The model under review builds one solid part; all positions refer to its coordinate system, in mm. Round coordinates to 2 decimals unless told otherwise and drop trailing zeros. Write each loop counter-clockwise with the first axis right and the second up, starting at its lowest first coordinate (ties: lowest second). Pieces come first, ordered by that corner, then holes. Notation, with made-up numbers: M -10.75,-17.75 L 23.25,-17.75 A21 ccw 23.25,12.25 Z; hole C 61.5,15.25 d8. An arc over 180 degrees is marked long. One line per item, written item: value. Start each with the question number.
1) Take a section at B-B, the plane x = 35. Write out the cut boundary in (y, z), and give its area (3 significant figures).
2) Take a section at A-A, the plane y = 12. Write out the cut boundary in (x, z), and give its area (3 significant figures).
3) Take a section at D-D, the plane z = 0. Write out the cut boundary in (x, y).
4) Take a section at C-C, the plane z = -35. Write out the cut boundary in (x, y).
5) For P1, Ø1, axis at x = -38.5, z = -12.5, coming from the +Y side; P2, Ø12, axis at y = 5, z = -22.5, coming from the +X side; P3, Ø12, axis at y = 13.5, z = -32, coming from the +X side, all flat-tipped, find the tip position at first contact; note any pin that passes through.
6) Wall thickness on probe 1 along Y at (x, z) = (41.5, -6.5); probe 2 along X at (y, z) = (5.5, -20); probe 3 along Z at (x, y) = (33, 16.5): over which ranges is each line inside the solid? List them lowest first.
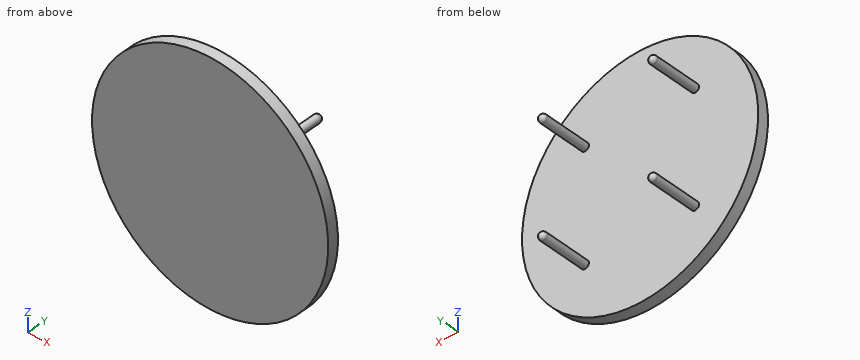
from build123d import *

# Parameters (mm, degrees)
SKETCH1_R                      = 75
BOSS_EXTRUDE1_DEPTH            = 7
SKETCH2_R                      = 2.5
BOSS_EXTRUDE2_DEPTH            = 30
DOME1_FACE_RADIUS              = 2.5
DOME1_HEIGHT                   = 2.5
CIRPATTERN1_COUNT              = 4
CIRPATTERN1_COPY_1_FACE_RADIUS = 2.5
CIRPATTERN1_COPY_1_HEIGHT      = 2.5
CIRPATTERN1_COPY_2_FACE_RADIUS = 2.5
CIRPATTERN1_COPY_2_HEIGHT      = 2.5
CIRPATTERN1_COPY_3_FACE_RADIUS = 2.5
CIRPATTERN1_COPY_3_HEIGHT      = 2.5


with BuildPart() as part:
    # Sketch1 → Boss-Extrude1 (new body)
    with BuildSketch(Plane(origin=(0, 0, 0), x_dir=(1, 0, 0), z_dir=(0, 1, 0))):
        with Locations(Location((0, 0, 0), (0, 0, 270))):
            Circle(SKETCH1_R)
    extrude(amount=BOSS_EXTRUDE1_DEPTH)

    # Sketch2 → Boss-Extrude2 (add)
    with BuildSketch(Plane(origin=(0, 7, 0), x_dir=(1, 0, 0), z_dir=(0, 1, 0))):
        with Locations(Location((35, 35, 0), (0, 0, 270))):
            Circle(SKETCH2_R)
    boss_extrude2 = extrude(amount=BOSS_EXTRUDE2_DEPTH)

    # Dome1: a dome of height H over a round flat face of radius A is a cap of a sphere of radius (A * A + H * H) / (2 * H)
    dome1_r = (DOME1_FACE_RADIUS * DOME1_FACE_RADIUS + DOME1_HEIGHT * DOME1_HEIGHT) / (2 * DOME1_HEIGHT)
    dome1_base = Plane((35, 37, -35), z_dir=(0, 1, 0))
    with Locations(dome1_base.offset(DOME1_HEIGHT - dome1_r)):
        dome1_ball = Sphere(dome1_r, mode=Mode.PRIVATE)
    add(split(dome1_ball, bisect_by=dome1_base, keep=Keep.TOP, mode=Mode.PRIVATE))

    # CirPattern1: Boss-Extrude2 ×4 about axis
    cirpattern1_axis = Axis((0, 0, 0), (0, 1, 0))
    for i in range(1, CIRPATTERN1_COUNT):
        add(boss_extrude2.rotate(cirpattern1_axis, i * 360 / CIRPATTERN1_COUNT))

    # CirPattern1 copy 1: a dome of height H over a round flat face of radius A is a cap of a sphere of radius (A * A + H * H) / (2 * H)
    cirpattern1_copy_1_r = (CIRPATTERN1_COPY_1_FACE_RADIUS * CIRPATTERN1_COPY_1_FACE_RADIUS + CIRPATTERN1_COPY_1_HEIGHT * CIRPATTERN1_COPY_1_HEIGHT) / (2 * CIRPATTERN1_COPY_1_HEIGHT)
    cirpattern1_copy_1_base = Plane((-35, 37, -35), z_dir=(0, 1, 0))
    with Locations(cirpattern1_copy_1_base.offset(CIRPATTERN1_COPY_1_HEIGHT - cirpattern1_copy_1_r)):
        cirpattern1_copy_1_ball = Sphere(cirpattern1_copy_1_r, mode=Mode.PRIVATE)
    add(split(cirpattern1_copy_1_ball, bisect_by=cirpattern1_copy_1_base, keep=Keep.TOP, mode=Mode.PRIVATE))

    # CirPattern1 copy 2: a dome of height H over a round flat face of radius A is a cap of a sphere of radius (A * A + H * H) / (2 * H)
    cirpattern1_copy_2_r = (CIRPATTERN1_COPY_2_FACE_RADIUS * CIRPATTERN1_COPY_2_FACE_RADIUS + CIRPATTERN1_COPY_2_HEIGHT * CIRPATTERN1_COPY_2_HEIGHT) / (2 * CIRPATTERN1_COPY_2_HEIGHT)
    cirpattern1_copy_2_base = Plane((-35, 37, 35), z_dir=(0, 1, 0))
    with Locations(cirpattern1_copy_2_base.offset(CIRPATTERN1_COPY_2_HEIGHT - cirpattern1_copy_2_r)):
        cirpattern1_copy_2_ball = Sphere(cirpattern1_copy_2_r, mode=Mode.PRIVATE)
    add(split(cirpattern1_copy_2_ball, bisect_by=cirpattern1_copy_2_base, keep=Keep.TOP, mode=Mode.PRIVATE))

    # CirPattern1 copy 3: a dome of height H over a round flat face of radius A is a cap of a sphere of radius (A * A + H * H) / (2 * H)
    cirpattern1_copy_3_r = (CIRPATTERN1_COPY_3_FACE_RADIUS * CIRPATTERN1_COPY_3_FACE_RADIUS + CIRPATTERN1_COPY_3_HEIGHT * CIRPATTERN1_COPY_3_HEIGHT) / (2 * CIRPATTERN1_COPY_3_HEIGHT)
    cirpattern1_copy_3_base = Plane((35, 37, 35), z_dir=(0, 1, 0))
    with Locations(cirpattern1_copy_3_base.offset(CIRPATTERN1_COPY_3_HEIGHT - cirpattern1_copy_3_r)):
        cirpattern1_copy_3_ball = Sphere(cirpattern1_copy_3_r, mode=Mode.PRIVATE)
    add(split(cirpattern1_copy_3_ball, bisect_by=cirpattern1_copy_3_base, keep=Keep.TOP, mode=Mode.PRIVATE))


solid = part.part
Checked values:
1. outline: M 0,-66.33 L 7,-66.33 L 7,-37.5 L 37,-37.5 A2.5 ccw 37,-32.5 L 7,-32.5 L 7,32.5 L 37,32.5 A2.5 ccw 37,37.5 L 7,37.5 L 7,66.33 L 0,66.33 Z
1. area: 1,250 mm2
2. outline: C -35,-35 d5; C -35,35 d5; C 35,-35 d5; C 35,35 d5
2. area: 78.5 mm2
3. outline: M -75,0 L 75,0 L 75,7 L -75,7 Z
4. outline: M -66.33,0 L 66.33,0 L 66.33,7 L 37.5,7 L 37.5,37 A2.5 ccw 32.5,37 L 32.5,7 L -32.5,7 L -32.5,37 A2.5 ccw -37.5,37 L -37.5,7 L -66.33,7 Z
5. P1: stops at y = 7
5. P2: stops at x = 73.16
5. P3: stops at x = 37.5
6. probe 1: y = 0 to 7
6. probe 2: x = -72.28 to 72.28
6. probe 3: z = -36.5 to -33.5, 33.5 to 36.5
